Source: three-view drawing plus pictorial views. Frame: mm from the lowest corner of the part. Coordinates: 2 decimals unless noted, no trailing zeros. Loops run counter-clockwise (first coordinate to the right, second up) from the corner with the lowest first, then second, coordinate; pieces in that order, holes last. Notation, with made-up numbers: M 63,83 L 68,83 A35 cw 68,116 Z; hole C 55.5,-34.5 d3. An arc over 180 degrees is marked long. Use a Markdown table: item, result. Add a question column.
1. Section A-A on y = 1.5. Output: boundary loops of the cut face in (x, z).
2. Section C-C on x = 9. Output: boundary loops of the cut face in (y, z) (1 decimal), then the cut area to 3 significant figures.
3. Section D-D on y = 5.5. Output: boundary loops of the cut face in (x, z), then the cut area to 3 significant figures.
4. Draft query along X for the marked faces 1, 2, 3 and 4. Return one class per face: +X half, -X half, draft (parallel to the pull), parting line (faces both ways), or undercut.
5. Section B-B on z = 4.75. Output: boundary loops of the cut face in (x, y) (1 decimal).
6. Line query: L1, parallel to Y at x = 6.5, z = 4.25; L2, parallel to Z at x = 7, y = 7.5 (1 decimal); L3, parallel to Z at x = 4.5, y = 7. Output: solid intervals per line, ascending. Write a range as [from, to].
7. Pin query (flat end, axial travel): pin 1 (2 mm diameter, centred on x = 3, y = 12, fed in from +Z) (1 decimal); pin 2 (1.5 mm diameter, centred on x = 6, y = 14, fed in from +Z); pin 3 (1.5 mm diameter, centred on y = 17, z = 7, fed in from +X). Return the tip coordinate at first contact, or that it passes through.
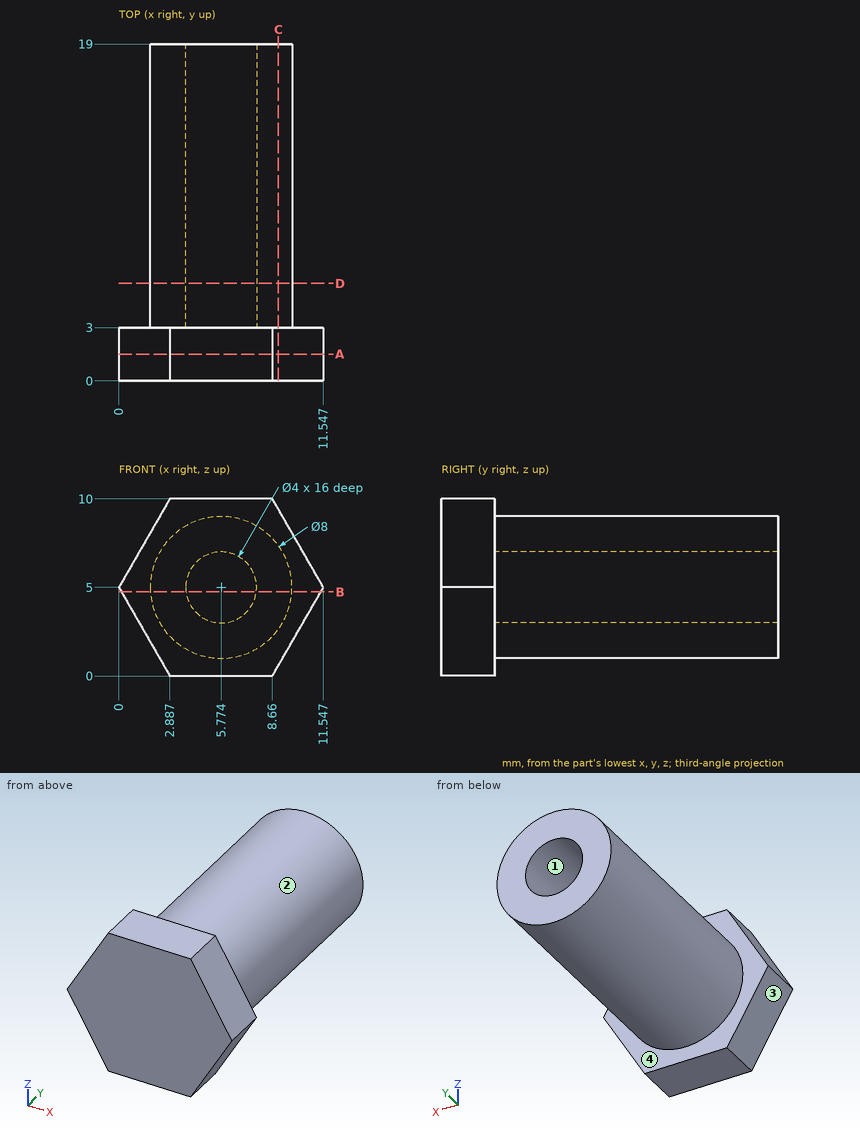
Answers below:
| question | item | result |
|---|---|---|
| 1 | outline | M 0,5 L 2.89,0 L 8.66,0 L 11.55,5 L 8.66,10 L 2.89,10 Z |
| 2 | outline | M 0,0.6 L 3,0.6 L 3,2.6 L 19,2.6 L 19,7.4 L 3,7.4 L 3,9.4 L 0,9.4 Z |
| 2 | area | 102 mm² |
| 3 | outline | C 5.77,5 d8; hole C 5.77,5 d4 |
| 3 | area | 37.7 mm² |
| 4 | face 1 | undercut |
| 4 | face 2 | parting line |
| 4 | face 3 | -X half |
| 4 | face 4 | draft |
| 5 | outline | M 0.1,0 L 11.4,0 L 11.4,3 L 9.8,3 L 9.8,19 L 7.8,19 L 7.8,3 L 3.8,3 L 3.8,19 L 1.8,19 L 1.8,3 L 0.1,3 Z |
| 6 | L1 | y = [0, 3] |
| 6 | L2 | z = [1.2, 3.4], [6.6, 8.8] |
| 6 | L3 | z = [1.21, 3.46], [6.54, 8.79] |
| 7 | pin 1 | stops at z = 8.6 |
| 7 | pin 2 | stops at z = 9 |
| 7 | pin 3 | stops at x = 9.57 |
